from build123d import *
from build123d.topology import SkipClean

# Parameters (mm, degrees)
CUT_EXTRUDE3_DEPTH      = 59.940648113
CUT_EXTRUDE3_DEPTH_BACK = 59.940648113
SKETCH3_W               = 17.579289035
SKETCH3_H               = 30.509322749
CUT_EXTRUDE4_DEPTH      = 59.268773799
CUT_EXTRUDE4_DEPTH_BACK = 59.268773799
SKETCH4_W               = 14.932737824
SKETCH4_H               = 19.875765969
CUT_EXTRUDE5_DEPTH      = 60.674114991
CUT_EXTRUDE5_DEPTH_BACK = 60.674114991
SKETCH5_R               = 5
CUT_EXTRUDE6_DEPTH      = 59.189346104
CUT_EXTRUDE6_DEPTH_BACK = 59.189346104
SKETCH6_W               = 15.994671042
SKETCH6_H               = 5.292782054
CUT_EXTRUDE7_DEPTH      = 58.976288256
CUT_EXTRUDE7_DEPTH_BACK = 25
SKETCH7_R               = 5


with BuildPart() as part:
    # Sketch1 → Revolve5 (revolve)
    with SkipClean():  # the faces are left unmerged after this step: merging them gives an invalid solid
        with BuildSketch(Plane.XY, mode=Mode.PRIVATE) as revolve5_sk:
            with BuildLine():
                ThreePointArc((10.5, 43), (7.424621202, 50.424621202), (0, 53.5))
                Line((0, 53.5), (0, 52.5))
                ThreePointArc((0, 52.5), (6.717514421, 49.717514421), (9.5, 43))
                ThreePointArc((9.5, 43), (6.717514421, 36.282485579), (0, 33.5))
                Line((0, 33.5), (0, 32.5))
                ThreePointArc((0, 32.5), (7.424621202, 35.575378798), (10.5, 43))
            make_face()
            with BuildLine():
                Line((0, 52.5), (0, 53.5))
                ThreePointArc((0, 53.5), (-10.5, 43), (0, 32.5))
                Line((0, 32.5), (0, 33.5))
                ThreePointArc((0, 33.5), (-9.5, 43), (0, 52.5))
            make_face()
        revolve(revolve5_sk.sketch.rotate(Axis((0, 0, 0), (0, 1, 0)), 180), axis=Axis((0, 0, 0), (0, 1, 0)))

    # Sketch1_7 → Revolve6 (revolve)
    with SkipClean():  # the faces are left unmerged after this step: merging them gives an invalid solid
        with BuildSketch(Plane.XY, mode=Mode.PRIVATE) as revolve6_sk:
            with BuildLine():
                Line((-7.5, 32.381619709), (-7.5, 4))
                Line((-7.5, 4), (-9, 4))
                Line((-9, 4), (-9, 0))
                Line((-9, 0), (0, 0))
                Line((0, 0), (0, 30))
                ThreePointArc((0, 30), (-3.934530227, 30.60970251), (-7.5, 32.381619709))
            make_face()
            with BuildLine():
                ThreePointArc((0, 56), (-12.39029749, 46.934530227), (-7.5, 32.381619709))
                ThreePointArc((-7.5, 32.381619709), (-3.934530227, 30.60970251), (0, 30))
                Line((0, 30), (0, 32.5))
                ThreePointArc((0, 32.5), (-10.5, 43), (0, 53.5))
                Line((0, 53.5), (0, 56))
            make_face()
            with BuildLine():
                ThreePointArc((13, 43), (9.192388155, 52.192388155), (0, 56))
                Line((0, 56), (0, 53.5))
                ThreePointArc((0, 53.5), (7.424621202, 50.424621202), (10.5, 43))
                ThreePointArc((10.5, 43), (7.424621202, 35.575378798), (0, 32.5))
                Line((0, 32.5), (0, 30))
                ThreePointArc((0, 30), (9.192388155, 33.807611845), (13, 43))
            make_face()
        revolve(revolve6_sk.sketch.rotate(Axis((0, 0, 0), (0, 1, 0)), 270), axis=Axis((0, 0, 0), (0, 1, 0)))

    # Sketch3 → Cut-Extrude3 (cut, two sides: drawn at the far end of the back side and taken through both)
    with SkipClean():  # the faces are left unmerged after this step: merging them gives an invalid solid
        with BuildSketch(Plane(origin=(0, 0, 0), x_dir=(0, 0, -1), z_dir=(1, 0, 0)).offset(-CUT_EXTRUDE3_DEPTH_BACK)):
            with Locations((-14.289644518, 47.636281084)):
                Rectangle(SKETCH3_W, SKETCH3_H)
            with Locations((14.289644518, 47.636281084)):
                Rectangle(SKETCH3_W, SKETCH3_H)
        extrude(amount=CUT_EXTRUDE3_DEPTH + CUT_EXTRUDE3_DEPTH_BACK, mode=Mode.SUBTRACT)

    # Sketch1_8 → Revolve7 (revolve)
    with SkipClean():  # the faces are left unmerged after this step: merging them gives an invalid solid
        with BuildSketch(Plane.XY, mode=Mode.PRIVATE) as revolve7_sk:
            with BuildLine():
                ThreePointArc((9.5, 43), (6.717514421, 49.717514421), (0, 52.5))
                Line((0, 52.5), (0, 33.5))
                ThreePointArc((0, 33.5), (6.717514421, 36.282485579), (9.5, 43))
            make_face()
            with BuildLine():
                Line((0, 33.5), (0, 52.5))
                ThreePointArc((0, 52.5), (-9.5, 43), (0, 33.5))
            make_face()
        revolve(revolve7_sk.sketch.rotate(Axis((0, 0, 0), (0, 1, 0)), 180), axis=Axis((0, 0, 0), (0, 1, 0)))

    # Sketch4 → Cut-Extrude4 (cut, two sides: drawn at the far end of the back side and taken through both)
    with BuildSketch(Plane(origin=(0, 0, 0), x_dir=(0, 0, -1), z_dir=(1, 0, 0)).offset(-CUT_EXTRUDE4_DEPTH_BACK)):
        with Locations((-14.466368912, 45.402031304)):
            Rectangle(SKETCH4_W, SKETCH4_H)
        with Locations((14.466368912, 45.402031304)):
            Rectangle(SKETCH4_W, SKETCH4_H)
    extrude(amount=CUT_EXTRUDE4_DEPTH + CUT_EXTRUDE4_DEPTH_BACK, mode=Mode.SUBTRACT)

    # Sketch5 → Cut-Extrude5 (cut, two sides: drawn at the far end of the back side and taken through both)
    with BuildSketch(Plane.XY.offset(7).offset(-CUT_EXTRUDE5_DEPTH_BACK)):
        with Locations((0, 43)):
            Circle(SKETCH5_R)
    extrude(amount=CUT_EXTRUDE5_DEPTH + CUT_EXTRUDE5_DEPTH_BACK, mode=Mode.SUBTRACT)

    # Sketch6 → Cut-Extrude6 (cut, two sides: drawn at the far end of the back side and taken through both)
    with BuildSketch(Plane(origin=(0, 0, 0), x_dir=(1, 0, 0), z_dir=(0, 1, 0)).offset(-CUT_EXTRUDE6_DEPTH_BACK)):
        with Locations((0.436218301, 10.146391027)):
            Rectangle(SKETCH6_W, SKETCH6_H)
        with Locations((0.436218301, -10.146391027)):
            Rectangle(SKETCH6_W, SKETCH6_H)
    extrude(amount=CUT_EXTRUDE6_DEPTH + CUT_EXTRUDE6_DEPTH_BACK, mode=Mode.SUBTRACT)

    # Sketch7 → Cut-Extrude7 (cut, two sides: drawn at the far end of the back side and taken through both)
    with BuildSketch(Plane.XZ.offset(-CUT_EXTRUDE7_DEPTH_BACK)):
        with Locations(Location((0, 0, 0), (0, 0, 90))):
            Circle(SKETCH7_R)
    extrude(amount=CUT_EXTRUDE7_DEPTH + CUT_EXTRUDE7_DEPTH_BACK, mode=Mode.SUBTRACT)


solid = part.part
Can you work these out from the model? Positions are in its coordinate system, mm. A direction names the side the tool comes from. Give positions to 0.01 mm unless a question says otherwise; leave off trailing zeros. Loops run counter-clockwise (first coordinate to the right, second up) from the corner with the lowest first, then second, coordinate; pieces in that order, holes last. Notation, with made-up numbers: (23, 18.25) - (72, 18.25) arc R19 cw to (72, 48.25) - close; hole circle Ø5 at (10.5, 77.25). An arc over 180 degrees is marked (long way). One line per item, written item: value.
(1) I need wall thicknesses on line 1 along X through (y, z) = (7.5, 0); line 2 along Y through (x, z) = (-0.75, 6.25); line 3 along Y through (x, z) = (0.75, 2). Which ranges of each line are inside material? Lowest first, please.
Verdict:
line 1: -7.5 to -5, 5 to 7.5
line 2: 0 to 32.38, 35.88 to 38.06, 47.94 to 50.12
line 3: 25 to 38.06, 47.94 to 55.82
(2) On a 3-axis mill with a long thin cutter (end or side, diameter ignored), from which of +Z, -Z, +X, -X, +Y, -Y can I reach the whole of each face in a straight line? I mean faces 1 (the face through (5.2, 43, 7)), 2 (the face through (-8, 4, -1)), 3 (the face through (8, 4, -1)), 4 (the face through (-9, 2, 0)), 5 (the face through (0, 51, 5.5)). Say none if no direction works.
Verdict:
face 1: +Z, +X, -X, +Y
face 2: -X
face 3: +X
face 4: -X, -Y
face 5: +Z
(3) I'm going to push flat-ended pins straight in: pin 1 (10.5 mm diameter, centred on x = -1, y = 44.5, fed in from +Z); pin 2 (8 mm diameter, centred on x = -3, z = -6, fed in from +Y); pin 3 (2 mm diameter, centred on x = -7.5, z = 4, fed in from +Y). Where does each tip first touch, or does it pass through?
Verdict:
pin 1: z = 7
pin 2: y = 55.71
pin 3: y = 53.62
(4) If we section it at B-B, the plane x = -2: List the corners of the cut face in (y, z) for me.
Verdict:
outline: (0, -7.5) - (4, -7.5) - (4, -7.23) - (32.38, -7.23) - (32.38, -5.5) - (35.52, -5.5) arc R9.29 ccw to (36.9, -7) - (38.42, -7) - (38.42, 7) - (36.9, 7) arc R9.29 ccw to (35.52, 5.5) - (32.38, 5.5) - (32.38, 7.23) - (4, 7.23) - (4, 7.5) - (0, 7.5) - (0, 4.58) - (25, 4.58) - (25, -4.58) - (0, -4.58) - close; (47.58, -7) - (49.1, -7) arc R9.29 ccw to (50.48, -5.5) - (54.61, -5.5) arc R12.85 ccw to (54.61, 5.5) - (50.48, 5.5) arc R9.29 ccw to (49.1, 7) - (47.58, 7) - close
(5) If we section it at C-C, the plane y = 15: List the corners of the cut face in (x, z) for me.
Verdict:
outline: circle Ø15 at (0, 0); hole circle Ø10 at (0, 0)
(6) If we section it at A-A, the plane z = 0: List the corners of the cut face in (x, y) for me, plus the area to 3 significant figures.
Verdict:
outline: (-9, 0) - (-5, 0) - (-5, 25) - (5, 25) - (5, 0) - (9, 0) - (9, 4) - (7.5, 4) - (7.5, 32.38) arc R13 ccw (long way) to (-7.5, 32.38) - (-7.5, 4) - (-9, 4) - close; hole circle Ø10 at (0, 43)
area: 676 mm^2
(7) If we section it at D-D, the plane z = -2.5: List the corners of the cut face in (x, y) for me, plus the area to 3 significant figures.
Verdict:
outline: (-8.65, 0) - (-4.33, 0) - (-4.33, 25) - (4.33, 25) - (4.33, 0) - (8.65, 0) - (8.65, 4) - (7.07, 4) - (7.07, 32.38) arc R12.76 ccw (long way) to (-7.07, 32.38) - (-7.07, 4) - (-8.65, 4) - close; hole circle Ø10 at (0, 43)
area: 666 mm^2
(8) If we mould it in two halves opening along X, with no side actions, what happens to faces 6 (the face through (0, 25, 0)), 7 (the face through (5.2, 43, -7)), 8 (the face through (-0.33, 17.992, 7.493))? For each: released by +X, released by -X, zero draft, split by the parting line, or undercut.
Verdict:
face 6: undercut
face 7: zero draft
face 8: split by the parting line
